Read the model definition and answer for the solid it produces. Units are mm, in the model's axes. Face numbers are marked on the shaded views. A direction names the side the tool comes from. Give positions to 0.01 mm unless a question says otherwise; leave off trailing zeros. Loops run counter-clockwise (first coordinate to the right, second up) from the corner with the lowest first, then second, coordinate; pieces in that order, holes last.
(1) Determine the mould class of the marked faces 4, 5 and 6 for opening direction X: pulls with the +X half, pulls with the -X half, needs draft (parallel to the pull), parting line crosses it, or undercut.
(2) Find section C-C, the plane y = -24.25. Write down the section's boundary in (x, z).
(3) Find section D-D, the plane x = 2.75. Write down the section's boundary in (y, z).
(4) Each of these flat-tipped pins is pushed along its axis until it touches: P1, Ø1, axis at x = 9.5, y = -24.5, coming from the -Z side; P2, Ø1.5, axis at y = -24.5, z = 9, coming from the +X side; P3, Ø6, axis at x = -9, y = -21.5, coming from the +Z side. Where does it stop, or does it pass through?
(5) Which of the six approach directions +Z, -Z, +X, -X, +Y, -Y give full straight-line access (tool end or side, diameter ignored) to the marked faces 1, 2 and 3?
(6) Straight lines are drawn through the part: probe 1 along Z at (x, y) = (-4.5, -27.5); probe 2 along Z at (x, y) = (1.75, -21.25); probe 3 along Y at (x, z) = (0, 14). For each, find the intervals that lie inside material, in ascending order.
(7) Find section A-A, the plane z = 11.43. Write down the section's boundary in (x, y).
(8) Find section B-B, the plane x = -1.5. Write down the section's boundary in (y, z), then the cut area to 3 significant figures.
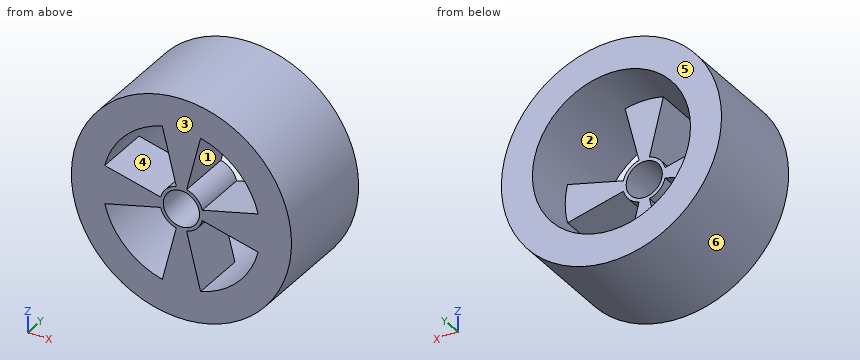
```python
from build123d import *

# Parameters (mm, degrees)
F2_R     = 2.032133
F3_DEPTH = 6.35


with BuildPart() as f1:
    # F0 (on Right) → F1 (revolve)
    with BuildSketch(Plane.YZ):
        Polygon((-29.244625, 23.807742), (-29.244625, 22.225), (-29.244625, 20.32), (-16.823784, 20.32), (-16.823784, 22.225), (-16.823784, 23.807742), align=None)
    revolve(axis=Axis((0, -22.716704, 11.43), (0, 1, 0)))

    # F2 (on face) → F3 (join)
    with BuildSketch(Plane.XZ.offset(29.244625)):
        with BuildLine():
            ThreePointArc((0.58379, 9.088548), (0, 9.016867), (-0.58379, 9.088548))
            Line((-0.58379, 9.088548), (-2.150686, 2.804071))
            ThreePointArc((-2.150686, 2.804071), (0, 2.54), (2.150686, 2.804071))
            Line((2.150686, 2.804071), (0.58379, 9.088548))
        make_face()
        with BuildLine():
            ThreePointArc((-2.341452, 10.84621), (-2.413133, 11.43), (-2.341452, 12.01379))
            Line((-2.341452, 12.01379), (-8.625929, 13.580686))
            ThreePointArc((-8.625929, 13.580686), (-8.89, 11.43), (-8.625929, 9.279314))
            Line((-8.625929, 9.279314), (-2.341452, 10.84621))
        make_face()
        with BuildLine():
            Line((-2.150686, 20.055929), (-0.58379, 13.771452))
            ThreePointArc((-0.58379, 13.771452), (0, 13.843133), (0.58379, 13.771452))
            Line((0.58379, 13.771452), (2.150686, 20.055929))
            ThreePointArc((2.150686, 20.055929), (0, 20.32), (-2.150686, 20.055929))
        make_face()
        with BuildLine():
            Line((8.625929, 13.580686), (2.341452, 12.01379))
            ThreePointArc((2.341452, 12.01379), (2.395146, 11.724087), (2.413133, 11.43))
            ThreePointArc((2.413133, 11.43), (2.395146, 11.135913), (2.341452, 10.84621))
            Line((2.341452, 10.84621), (8.625929, 9.279314))
            ThreePointArc((8.625929, 9.279314), (8.823735, 10.346582), (8.89, 11.43))
            ThreePointArc((8.89, 11.43), (8.823735, 12.513418), (8.625929, 13.580686))
        make_face()
        with BuildLine():
            ThreePointArc((0.58379, 13.771452), (0, 13.843133), (-0.58379, 13.771452))
            ThreePointArc((-0.58379, 13.771452), (-1.706342, 13.136342), (-2.341452, 12.01379))
            ThreePointArc((-2.341452, 12.01379), (-2.413133, 11.43), (-2.341452, 10.84621))
            ThreePointArc((-2.341452, 10.84621), (-1.706342, 9.723658), (-0.58379, 9.088548))
            ThreePointArc((-0.58379, 9.088548), (0, 9.016867), (0.58379, 9.088548))
            ThreePointArc((0.58379, 9.088548), (1.706342, 9.723658), (2.341452, 10.84621))
            ThreePointArc((2.341452, 10.84621), (2.395146, 11.135913), (2.413133, 11.43))
            ThreePointArc((2.413133, 11.43), (2.395146, 11.724087), (2.341452, 12.01379))
            ThreePointArc((2.341452, 12.01379), (1.706342, 13.136342), (0.58379, 13.771452))
        make_face()
        with Locations((0, 11.43)):
            Circle(F2_R, mode=Mode.SUBTRACT)
    extrude(amount=-F3_DEPTH)


solid = f1.part
```
Entries:
1. face 4: undercut
1. face 5: needs draft
1. face 6: parting line crosses it
2. outline: circle Ø24.76 at (0, 11.43); hole (-8.63, 9.28) arc R8.89 ccw to (-2.15, 2.8) - (-0.58, 9.09) arc R2.41 cw to (-2.34, 10.85) - close; hole (-8.63, 13.58) - (-2.34, 12.01) arc R2.41 cw to (-0.58, 13.77) - (-2.15, 20.06) arc R8.89 ccw to start; hole circle Ø4.06 at (0, 11.43); hole (0.58, 9.09) - (2.15, 2.8) arc R8.89 ccw to (8.63, 9.28) - (2.34, 10.85) arc R2.41 cw to start; hole (0.58, 13.77) arc R2.41 cw to (2.34, 12.01) - (8.63, 13.58) arc R8.89 ccw to (2.15, 20.06) - close
3. outline: (-29.24, -0.64) - (-16.82, -0.64) - (-16.82, 2.98) - (-29.24, 2.98) - close; (-29.24, 10.74) - (-22.89, 10.74) - (-22.89, 12.12) - (-29.24, 12.12) - close; (-29.24, 19.88) - (-16.82, 19.88) - (-16.82, 23.5) - (-29.24, 23.5) - close
4. P1: stops at z = 2.93
4. P2: stops at x = 12.26
4. P3: stops at z = 22.26
5. face 1: +Y, -Y
5. face 2: +Y
5. face 3: +Z, -Z, +X, -X, -Y
6. probe 1: z = -0.1 to 3.76, 10.31 to 12.55, 19.1 to 22.96
6. probe 2: z = -0.82 to 2.71, 20.15 to 23.68
6. probe 3: y = -29.24 to -22.89
7. outline: (-12.38, -29.24) - (-2.03, -29.24) - (-2.03, -22.89) - (-8.89, -22.89) - (-8.89, -16.82) - (-12.38, -16.82) - close; (2.03, -29.24) - (12.38, -29.24) - (12.38, -16.82) - (8.89, -16.82) - (8.89, -22.89) - (2.03, -22.89) - close
8. outline: (-29.24, -0.86) - (-16.82, -0.86) - (-16.82, 2.67) - (-22.89, 2.67) - (-22.89, 5.41) - (-29.24, 5.41) - close; (-29.24, 9.54) - (-22.89, 9.54) - (-22.89, 10.06) - (-29.24, 10.06) - close; (-29.24, 12.8) - (-22.89, 12.8) - (-22.89, 13.32) - (-29.24, 13.32) - close; (-29.24, 17.45) - (-22.89, 17.45) - (-22.89, 20.19) - (-16.82, 20.19) - (-16.82, 23.72) - (-29.24, 23.72) - close
8. area: 129 mm2
